Input: dimensioned drawing with shaded views. Units: mm. Origin: part minimum x, y, z. A direction names the side the tool comes from. Give positions to 0.01 mm unless a question says otherwise; leave off trailing zeros. Order: outer loops, then holes, each group sorted by start corner. A loop starts at its lowest first (then second) coordinate and runs counter-clockwise, first axis right, second up. Notation, with made-up numbers: M 45.25,83 L 89.25,83 A13 cw 89.25,97 Z; hole C 66,-30 d3. An arc over 180 degrees is marked long. Answer in a Markdown table with one row per item. Add a question column.
(1) Section query A-A, the plane y = 12. Return loops of the section in (x, z) (1 decimal), plus the area to 3 significant figures.
(2) Pin query (flat end, axial travel): P1, Ø11.5, axis at x = 117, z = 15.5, coming from the +Y side; P2, Ø4, axis at y = 10, z = 12.5, coming from the -X side; P3, Ø12, axis at y = 8.5, z = 5.5, coming from the +X side. Return the tip coordinate at first contact, or that it passes through.
(3) Set-up query: the marked faces 1, 2 and 3. Return all of +Z, -Z, +X, -X, +Y, -Y with unobstructed straight access to the full face (end or side cutting, diameter ignored); none if empty.
(4) Material intervals for line 1 along X through (y, z) = (8.25, 20) (1 decimal); line 2 along Z through (x, y) = (29.5, 9) (1 decimal); line 3 along X through (y, z) = (8.25, 2.5) (1 decimal), sorted ascending.
(5) Section query B-B, the plane z = 17. Return loops of the section in (x, y) (1 decimal), plus the area to 3 significant figures.
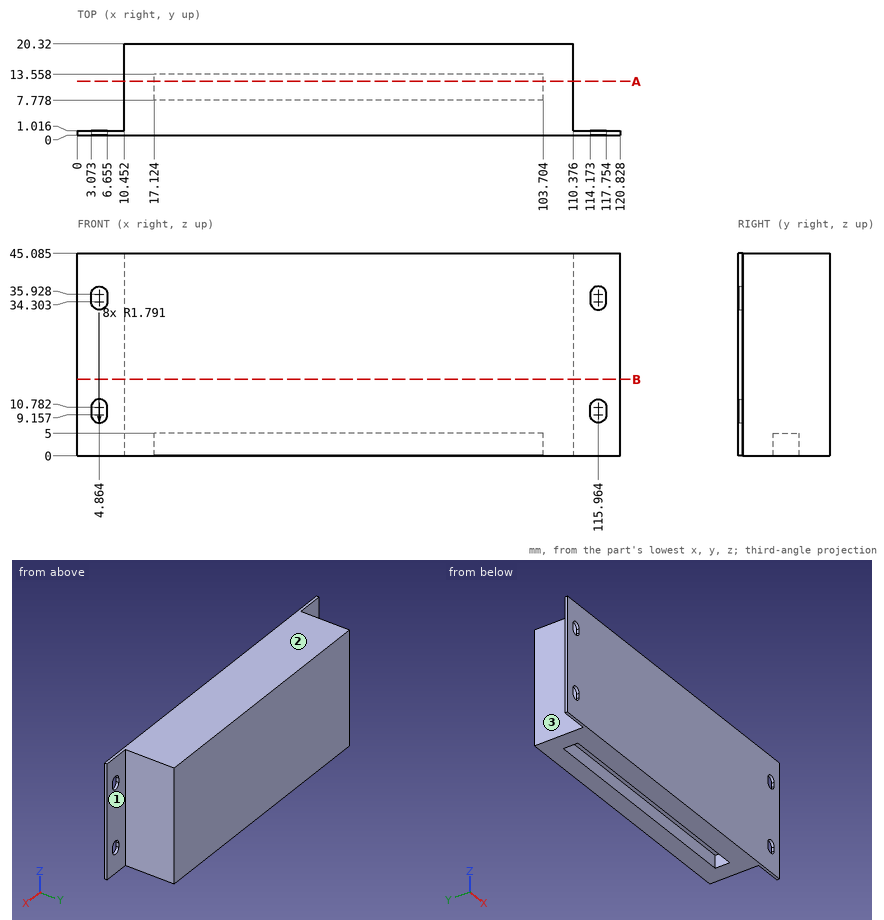
Values follow:
| question | item | result |
|---|---|---|
| 1 | outline | M 10.5,0 L 17.1,0 L 17.1,5 L 103.7,5 L 103.7,0 L 110.4,0 L 110.4,45.1 L 10.5,45.1 Z |
| 1 | area | 4,070 mm² |
| 2 | P1 | stops at y = 1.02 |
| 2 | P2 | stops at x = 10.45 |
| 2 | P3 | stops at x = 110.38 |
| 3 | face 1 | +Z, -Z, +X, +Y |
| 3 | face 2 | +Z, +X, -X, +Y, -Y |
| 3 | face 3 | +Z, -Z, -X, +Y |
| 4 | line 1 | x = 10.5 to 110.4 |
| 4 | line 2 | z = 5 to 45.1 |
| 4 | line 3 | x = 10.5 to 17.1, 103.7 to 110.4 |
| 5 | outline | M 0,0 L 120.8,0 L 120.8,1 L 110.4,1 L 110.4,20.3 L 10.5,20.3 L 10.5,1 L 0,1 Z |
| 5 | area | 2,050 mm² |
